```python
from build123d import *

# Parameters (mm, degrees)
SKETCH1_R            = 3
BOSS_EXTRUDE1_DEPTH  = 40
SKETCH2_W            = 32
SKETCH2_H            = 50
BOSS_EXTRUDE2_DEPTH  = 20
SKETCH9_W            = 48
SKETCH9_H            = 20
BOSS_EXTRUDE5_DEPTH  = 4
FILLET1_R            = 2
SKETCH10_W           = 24
SKETCH10_H           = 20
CUT_EXTRUDE2_DEPTH   = 18
SKETCH11_W           = 5
SKETCH11_H           = 3.5
CUT_EXTRUDE3_DEPTH   = 5
FILLET1_OF_MIRROR5_R = 2


with BuildPart() as part:
    # Sketch1 → Boss-Extrude1 (new, symmetric)
    with BuildSketch(Plane.XY):
        Circle(SKETCH1_R)
    extrude(amount=BOSS_EXTRUDE1_DEPTH, both=True)

    # Sketch2 → Boss-Extrude2 (add)
    with BuildSketch(Plane.XY.offset(40)):
        Rectangle(SKETCH2_W, SKETCH2_H)
    boss_extrude2 = extrude(amount=BOSS_EXTRUDE2_DEPTH)

    # Sketch9 → Boss-Extrude5 (add)
    with BuildSketch(Plane.XZ.offset(25)):
        with Locations((0, 50)):
            Rectangle(SKETCH9_W, SKETCH9_H)
    boss_extrude5 = extrude(amount=-BOSS_EXTRUDE5_DEPTH)

    # Fillet1
    fillet1_edges = [part.edges().sort_by_distance(p)[0] for p in [
        (-16, -21, 50),
        (16, -21, 50),
    ]]
    fillet(fillet1_edges, radius=FILLET1_R)

    # Sketch10 → Cut-Extrude2 (cut)
    with BuildSketch(Plane(origin=(0, 25, 0), x_dir=(1, 0, 0), z_dir=(0, 1, 0))):
        with Locations((0, -50)):
            Rectangle(SKETCH10_W, SKETCH10_H)
    cut_extrude2 = extrude(amount=-CUT_EXTRUDE2_DEPTH, mode=Mode.SUBTRACT)

    # Sketch11 → Cut-Extrude3 (cut)
    with BuildSketch(Plane(origin=(0, 7, 0), x_dir=(1, 0, 0), z_dir=(0, 1, 0))):
        with Locations((0, -50)):
            Rectangle(SKETCH11_W, SKETCH11_H)
    cut_extrude3 = extrude(amount=-CUT_EXTRUDE3_DEPTH, mode=Mode.SUBTRACT)

    # Mirror5: Boss-Extrude2, Boss-Extrude5, Cut-Extrude2, Cut-Extrude3 across plane
    add(boss_extrude2.mirror(Plane.XY))
    add(boss_extrude5.mirror(Plane.XY))
    add(cut_extrude2.mirror(Plane.XY), mode=Mode.SUBTRACT)
    add(cut_extrude3.mirror(Plane.XY), mode=Mode.SUBTRACT)

    # Fillet1 of Mirror5
    fillet1_of_mirror5_edges = [part.edges().sort_by_distance(p)[0] for p in [
        (-16, -21, -50),
        (16, -21, -50),
    ]]
    fillet(fillet1_of_mirror5_edges, radius=FILLET1_OF_MIRROR5_R)


solid = part.part
```
Read the model definition and answer for the solid it produces. Units are mm, in the model's axes. A direction names the side the tool comes from. Give positions to 0.01 mm unless a question says otherwise; leave off trailing zeros. Order: outer loops, then holes, each group sorted by start corner. A loop starts at its lowest first (then second) coordinate and runs counter-clockwise, first axis right, second up. Notation, with made-up numbers: (-20.75, 86.5) -> (0.25, 86.5) arc R28 ccw to (0.25, 115.5) -> close; hole circle Ø9 at (73.25, 3.5). An arc over 180 degrees is marked (long way). One line per item, written item: value. Start each with the question number.
(1) The part is cut by section A-A (x = 9.5). Determine the outline of the cut face in (y, z).
(2) The part is cut by section C-C (y = -15.5). Determine the outline of the cut face in (x, z), and give its area (3 significant figures).
(3) A tool of negligible diameter and unlimited length cuts with its end or side. For faces 1 (the flat face through (-16, 3, 50)), 2 (the flat face through (-2.5, 5, 50)), 3 (the flat face through (0, 7, 48)), from which of +Z, -Z, +X, -X, +Y, -Y can it reach the whole face along a straight path? Write none if from no direction.
(4) The part is cut by section D-D (x = 0). Determine the outline of the cut face in (y, z).
(5) Straight lines are drawn through the part: L1, parallel to Z at x = 15, y = -5; L2, parallel to Y at x = 10, z = 54.5; L3, parallel to Y at x = 19, z = -49.5. For each, find the intervals that lie inside material, in ascending order.
(6) Flat-ended cylindrical pins translate along their axes: P1, Ø6, axis at y = 4.5, z = -54.5, coming from the -X side; P2, Ø3, axis at x = 22, z = 50, coming from the +Y side; P3, Ø16, axis at y = 2.5, z = -54.5, coming from the +X side. Find the tip coordinate at first contact, or state that the pin passes through.
(7) The part is cut by section B-B (y = 13). Determine the outline of the cut face in (x, z).
(8) For a pull along X with two mould halves and no side action, classify faces 4 (the flat face through (0, 2, -50)), 5 (the flat face through (-2.5, 5, -50)), 6 (the flat face through (-16, 3, -50)), 7 (the flat face through (14, 25, -50)) as released by +X, released by -X, zero draft, split by the parting line, or undercut.
Taken from the geometry:
1. outline: (-25, -60) -> (7, -60) -> (7, -40) -> (-25, -40) -> close; (-25, 40) -> (7, 40) -> (7, 60) -> (-25, 60) -> close
2. outline: (-16, -60) -> (16, -60) -> (16, -40) -> (-16, -40) -> close; (-16, 40) -> (16, 40) -> (16, 60) -> (-16, 60) -> close
2. area: 1,280 mm^2
3. face 1: +Z, -Z, -X, +Y
3. face 2: +Y
3. face 3: +Z, -Z, +Y
4. outline: (-25, -60) -> (7, -60) -> (7, -51.75) -> (2, -51.75) -> (2, -48.25) -> (7, -48.25) -> (7, -40) -> (3, -40) -> (3, 40) -> (7, 40) -> (7, 48.25) -> (2, 48.25) -> (2, 51.75) -> (7, 51.75) -> (7, 60) -> (-25, 60) -> (-25, 40) -> (-3, 40) -> (-3, -40) -> (-25, -40) -> close
5. L1: -60 to -40, 40 to 60
5. L2: -25 to 7
5. L3: -25 to -21
6. P1: x = -16
6. P2: y = -21
6. P3: x = 16
7. outline: (-16, -60) -> (-12, -60) -> (-12, -40) -> (-16, -40) -> close; (-16, 40) -> (-12, 40) -> (-12, 60) -> (-16, 60) -> close; (12, -60) -> (16, -60) -> (16, -40) -> (12, -40) -> close; (12, 40) -> (16, 40) -> (16, 60) -> (12, 60) -> close
8. face 4: undercut
8. face 5: undercut
8. face 6: released by -X
8. face 7: zero draft
